Could you check a few things on this drawing? It's one solid part, dimensions in mm from its lowest x, y, z. Give positions to 0.01 mm unless a question says otherwise; leave off trailing zeros. Loops run counter-clockwise (first coordinate to the right, second up) from the corner with the lowest first, then second, coordinate; pieces in that order, holes last. Notation, with made-up numbers: (-36, 38) - (-27, 38) arc R35 cw to (-27, 75) - close; hole circle Ø8 at (11, -9.75). An arc over 180 degrees is marked (long way). Return JSON: item names as keys, results as strings. Group by question number.
(1) For P1, Ø1, axis at x = 2, z = 7, coming from the -Y side (3 decimals), with a flat end and sliding along its axis, tell me the tip position at first contact or that it passes through.
(2) I need wall thicknesses on probe 1 along Z at (x, y) = (7, 13); probe 2 along X at (y, z) = (144.02, 0.55); probe 3 along X at (y, z) = (58.5, 2.25). Which ranges of each line are inside material? Lowest first, please. Write a range as [from, to].
(3) If we section it at B-B (x = 12.5): Please give me the cut outline in (y, z), then the cut area to 3 significant figures.
(4) If we section it at A-A (z = 4): Please give me the cut outline in (x, y).
(5) If we section it at D-D (y = 144.02): Please give me the cut outline in (x, z).
(6) If we section it at C-C (y = 41): Please give me the cut outline in (x, z).
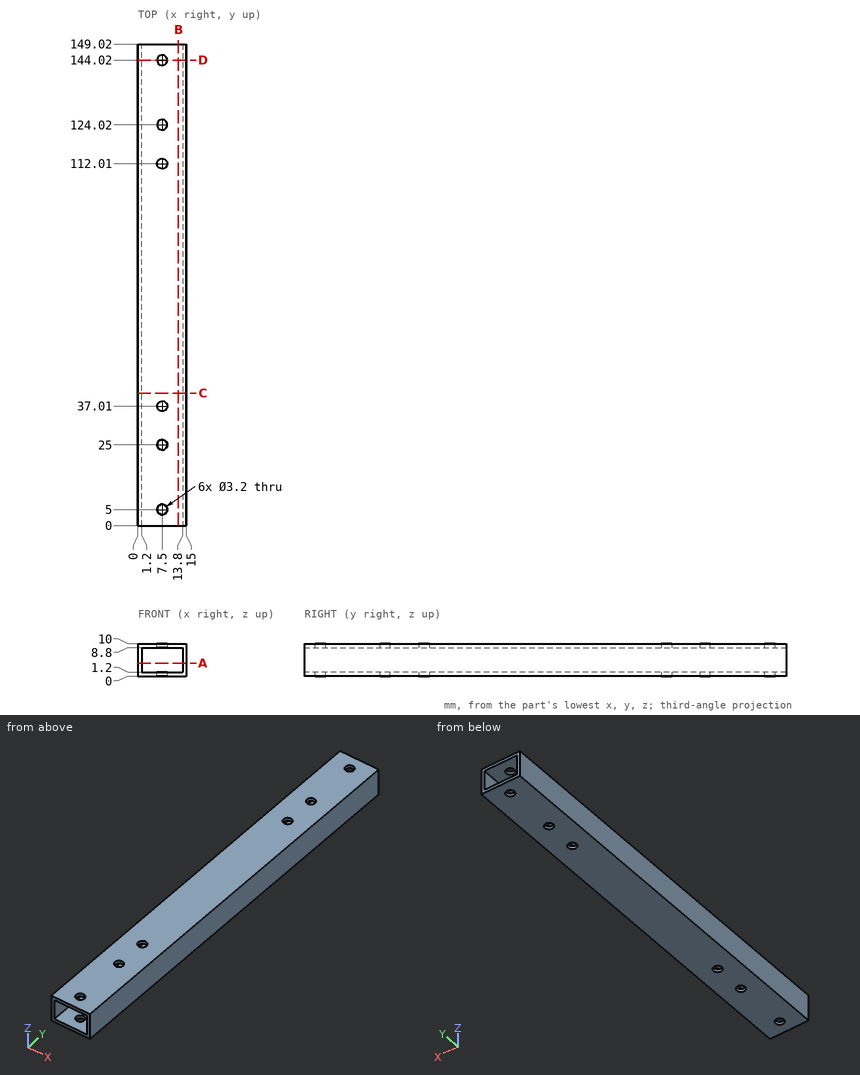
Values:
{
 "1": {"P1": "through"},
 "2": {"probe 1": "[0, 1.2], [8.8, 10]", "probe 2": "[0, 5.9], [9.1, 15]", "probe 3": "[0, 1.2], [13.8, 15]"},
 "3": {"outline": "(0, 0) - (149.02, 0) - (149.02, 1.2) - (0, 1.2) - close; (0, 8.8) - (149.02, 8.8) - (149.02, 10) - (0, 10) - close", "area": "358 mm2"},
 "4": {"outline": "(0, 0) - (1.2, 0) - (1.2, 149.02) - (0, 149.02) - close; (13.8, 0) - (15, 0) - (15, 149.02) - (13.8, 149.02) - close"},
 "5": {"outline": "(0, 0) - (5.9, 0) - (5.9, 1.2) - (1.2, 1.2) - (1.2, 8.8) - (5.9, 8.8) - (5.9, 10) - (0, 10) - close; (9.1, 0) - (15, 0) - (15, 10) - (9.1, 10) - (9.1, 8.8) - (13.8, 8.8) - (13.8, 1.2) - (9.1, 1.2) - close"},
 "6": {"outline": "(0, 0) - (15, 0) - (15, 10) - (0, 10) - close; hole (1.2, 1.2) - (13.8, 1.2) - (13.8, 8.8) - (1.2, 8.8) - close"}
}
